Read the model definition and answer for the solid it produces. Units are mm, in the model's axes. Round coordinates to 2 decimals unless told otherwise and drop trailing zeros. Write each loop counter-clockwise with the first axis right and the second up, starting at its lowest first coordinate (ties: lowest second). Pieces come first, ordered by that corner, then holes.
from build123d import *

# Parameters (mm, degrees)
SKETCH1_W           = 115
SKETCH1_H           = 38.1
BOSS_EXTRUDE1_DEPTH = 1.016
CUT_EXTRUDE2_DEPTH  = 61.582049784


with BuildPart() as part:
    # Sketch1 → Boss-Extrude1 (new body)
    with BuildSketch(Plane.XY):
        Rectangle(SKETCH1_W, SKETCH1_H)
    extrude(amount=BOSS_EXTRUDE1_DEPTH)

    # Sketch2 → Cut-Extrude2 (cut, through all)
    with BuildSketch(Plane.XY):
        Polygon((-57.5, 19.05), (-57.5, -19.05), (-43.921959921, -19.05), align=None)
        Polygon((57.5, -19.05), (57.5, 19.05), (43.921959921, -19.05), align=None)
        with BuildLine():
            ThreePointArc((-1.524320269, 7.904362604), (0, -8.050000029), (1.524320269, 7.904362604))
            ThreePointArc((1.524320269, 7.904362604), (0, 9.475003402), (-1.524320269, 7.904362604))
        make_face()
    extrude(amount=CUT_EXTRUDE2_DEPTH, mode=Mode.SUBTRACT)


solid = part.part
Q1. Straight lines are drawn through the part: probe 1 along Y at (x, z) = (0, 0.6) (3 decimals); probe 2 along X at (y, z) = (0, 0.15); probe 3 along X at (y, z) = (7, 0.3). For each, find the intervals that lie inside material, in ascending order.
Verdict:
probe 1: y = -19.05 to -8.05, 9.475 to 19.05
probe 2: x = -50.71 to -8.05, 8.05 to 50.71
probe 3: x = -53.21 to -3.98, 3.98 to 53.21
Q2. Section B-B (y = 0) is taken. Determine the outline of the cut face in (x, z), then the cut area to 3 significant figures.
Verdict:
outline: (-50.71, 0) - (-8.05, 0) - (-8.05, 1.02) - (-50.71, 1.02) - close; (8.05, 0) - (50.71, 0) - (50.71, 1.02) - (8.05, 1.02) - close
area: 86.7 mm2
Q3. Determine the mould class of faces 1 (the flat face through (-50.616, -0.267, 0.501)), 2 (the flat face through (-0.8, -8.2, 1.016)), 3 (the cylindrical face through (-0.332, -8.043, 0.501)), 4 (the flat face through (50.806, 0.267, 0.501)) for opening direction X: pulls with the +X half, pulls with the -X half, needs draft (parallel to the pull), parting line crosses it, or undercut.
Verdict:
face 1: pulls with the -X half
face 2: needs draft
face 3: undercut
face 4: pulls with the +X half
Q4. Section A-A (x = 0) is taken. Determine the outline of the cut face in (y, z) (3 decimals), then the cut area to 3 significant figures.
Verdict:
outline: (-19.05, 0) - (-8.05, 0) - (-8.05, 1.016) - (-19.05, 1.016) - close; (9.475, 0) - (19.05, 0) - (19.05, 1.016) - (9.475, 1.016) - close
area: 20.9 mm2
Q5. Section C-C (z = 0.85) is taken. Determine the outline of the cut face in (x, y) (3 decimals), then the cut area to 3 significant figures.
Verdict:
outline: (-57.5, 19.05) - (-43.922, -19.05) - (43.922, -19.05) - (57.5, 19.05) - close; hole (-1.524, 7.904) arc R8.05 ccw (long way) to (1.524, 7.904) arc R1.525 ccw (long way) to start
area: 3,660 mm2
